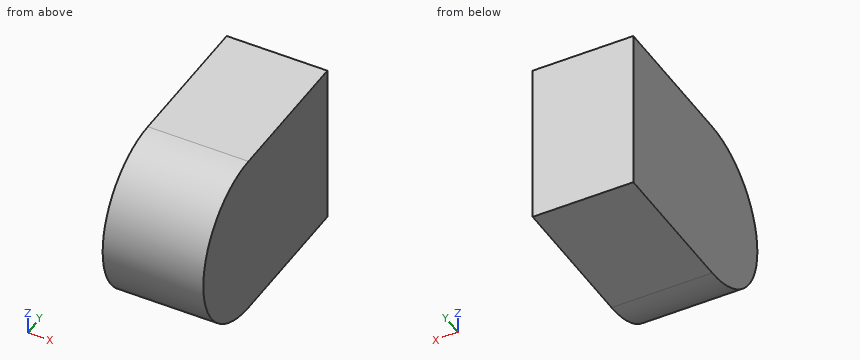
from build123d import *

# Parameters (mm, degrees)
EXTRUDE_1_DEPTH = 1
EXTRUDE_2_DEPTH = 14.6
EXTRUDE_3_DEPTH = 6
EXTRUDE_4_DEPTH = 2.5
EXTRUDE_6_DEPTH = 2.7


with BuildPart() as part:
    # 草图1 → 凸台-拉伸1 (new body)
    with BuildSketch(Plane(origin=(0, 0, 0), x_dir=(0, 0, -1), z_dir=(1, 0, 0))):
        with BuildLine():
            Line((15, 0), (15, 26.2))
            Line((15, 26.2), (-15, 26.2))
            Line((-15, 26.2), (-15, 0))
            ThreePointArc((-15, 0), (0, -15), (15, 0))
        make_face()
    extrude(amount=EXTRUDE_1_DEPTH)

    # 草图2 → 凸台-拉伸2 (add)
    with BuildSketch(Plane(origin=(1, 0, 0), x_dir=(0, 0, -1), z_dir=(1, 0, 0))):
        with BuildLine():
            Line((15, 0), (15, 26.2))
            Line((15, 26.2), (-15, 26.2))
            Line((-15, 26.2), (-15, 0))
            ThreePointArc((-15, 0), (0, -15), (15, 0))
        make_face()
        with BuildLine():
            Line((14, 0), (14, 25.2))
            Line((14, 25.2), (-14, 25.2))
            Line((-14, 25.2), (-14, 0))
            ThreePointArc((-14, 0), (0, -14), (14, 0))
        make_face(mode=Mode.SUBTRACT)
    extrude(amount=EXTRUDE_2_DEPTH)

    # 草图4 → 凸台-拉伸3 (add)
    with BuildSketch(Plane(origin=(3.6, 0, 0), x_dir=(0, 0, -1), z_dir=(1, 0, 0))):
        Polygon((8.5, 8.7), (14, 14.2), (14, 20.2), (-14, 20.2), (-14, 14.2), (-8.5, 8.7), align=None)
    extrude(amount=EXTRUDE_3_DEPTH)

    # 草图5 → 凸台-拉伸4 (add)
    with BuildSketch(Plane(origin=(14.6, 0, 0), x_dir=(0, 0, -1), z_dir=(1, 0, 0))):
        Polygon((14, 14.2), (14, 20.2), (-14, 20.2), (-14, 14.2), (-8.5, 8.7), (8.5, 8.7), align=None)
    extrude(amount=-EXTRUDE_4_DEPTH)

    # 草图6 → 凸台-拉伸6 (add)
    with BuildSketch(Plane(origin=(15.6, 0, 0), x_dir=(0, 0, -1), z_dir=(1, 0, 0))):
        with BuildLine():
            Line((-15, 0), (-15, 26.2))
            Line((-15, 26.2), (15, 26.2))
            Line((15, 26.2), (15, 0))
            ThreePointArc((15, 0), (0, -15), (-15, 0))
        make_face()
    extrude(amount=EXTRUDE_6_DEPTH)


solid = part.part
CAD build for the part. Positions are in the model's coordinates, mm. Round coordinates to 2 decimals unless told otherwise and drop trailing zeros. Loops run counter-clockwise (first coordinate to the right, second up) from the corner with the lowest first, then second, coordinate; pieces in that order, holes last. Notation, with made-up numbers: M 46.25,25 L 88.25,25 A14 ccw 88.25,41 Z; hole C 66,-37 d10. An arc over 180 degrees is marked long. One line per question, with ' | ' between items. Start each with the question number.
Item 1: Wall check: line 1 (X direction, y = 10, z = -5.5); line 2 (Z direction, x = 8.25, y = 0.5); line 3 (X direction, y = 24.5, z = 6). Give the ranges that are in metal, low to high.
Item 2: Cut at C-C, the plane y = 21.5. Write the cut outline in (x, z), plus the area to 3 significant figures.
Item 3: Cut at D-D, the plane z = -5. Write the cut outline in (x, y), plus the area to 3 significant figures.
Item 4: Pin check, flat tips, straight feed: pin 1 Ø1.5 at (x, y) = (3.5, -3.5) entering from -Z; pin 2 Ø12.5 at (y, z) = (15, 3.5) entering from -X; pin 3 Ø1.2 at (x, z) = (13, -4) entering from -Y; pin 4 Ø8 at (x, y) = (6, -7) entering from +Z. Stop position of each tip, or through.
Item 5: Cut at B-B, the plane x = 7. Write the cut outline in (y, z), plus the area to 3 significant figures.
Item 6: Cut at A-A, the plane z = 0. Write the cut outline in (x, y), plus the area to 3 significant figures.
Responses:
1) line 1: x = 0 to 1, 3.6 to 9.6, 12.1 to 14.6, 15.6 to 18.3 | line 2: z = -15 to -14, 14 to 15 | line 3: x = 0 to 1, 15.6 to 18.3
2) outline: M 0,-15 L 18.3,-15 L 18.3,15 L 0,15 Z; hole M 1,-14 L 15.6,-14 L 15.6,14 L 1,14 Z | area: 140 mm²
3) outline: M 0,-14.14 L 18.3,-14.14 L 18.3,26.2 L 0,26.2 Z; M 3.6,8.7 L 9.6,8.7 L 9.6,20.2 L 3.6,20.2 Z; M 12.1,8.7 L 14.6,8.7 L 14.6,20.2 L 12.1,20.2 Z; hole M 1,-13.08 L 15.6,-13.08 L 15.6,25.2 L 1,25.2 Z | area: 277 mm²
4) pin 1: stops at z = -14.75 | pin 2: stops at x = 0 | pin 3: stops at y = -14.61 | pin 4: stops at z = 14.7
5) outline: M 0,-15 L 26.2,-15 L 26.2,15 L 0,15 A15 ccw Z; hole M 0,-14 L 14.2,-14 L 8.7,-8.5 L 8.7,8.5 L 14.2,14 L 0,14 A14 ccw Z; hole M 20.2,-14 L 25.2,-14 L 25.2,14 L 20.2,14 Z | area: 418 mm²
6) outline: M 0,-15 L 18.3,-15 L 18.3,26.2 L 0,26.2 Z; M 3.6,8.7 L 9.6,8.7 L 9.6,20.2 L 3.6,20.2 Z; M 12.1,8.7 L 14.6,8.7 L 14.6,20.2 L 12.1,20.2 Z; hole M 1,-14 L 15.6,-14 L 15.6,25.2 L 1,25.2 Z | area: 279 mm²
